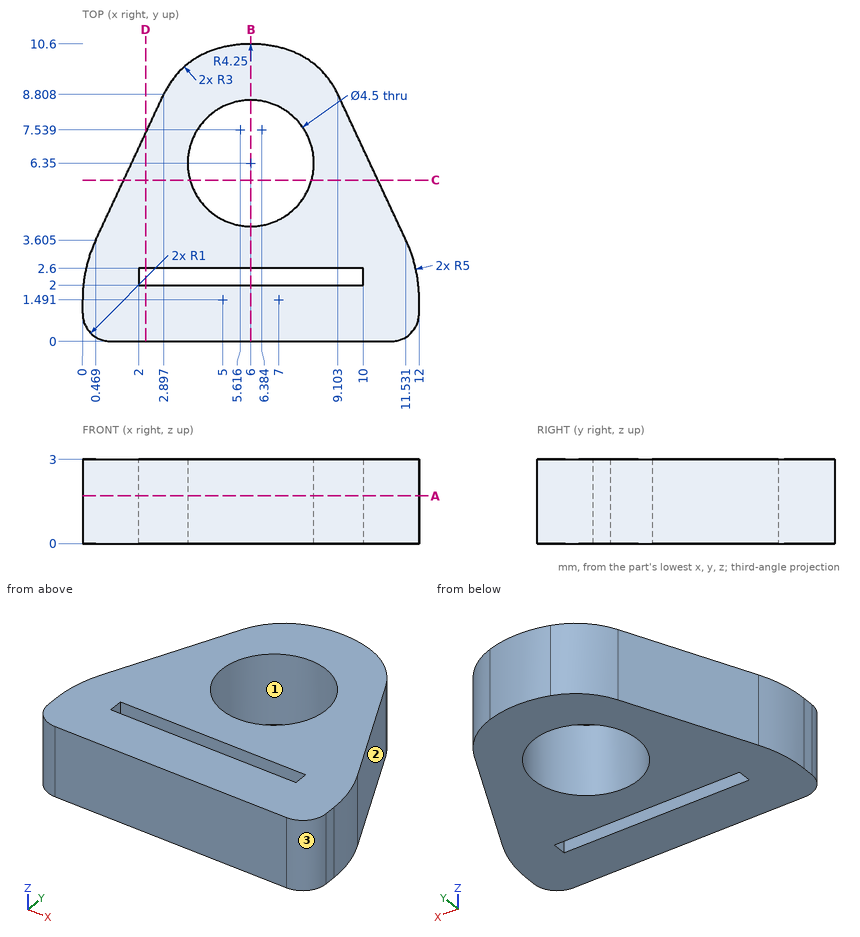
The drawing under review shows one solid part. Ordinate dimensions are in mm from its lowest x, y, z. Give positions to 0.01 mm unless a question says otherwise; leave off trailing zeros. Write each loop counter-clockwise with the first axis right and the second up, starting at its lowest first coordinate (ties: lowest second). Pieces come first, ordered by that corner, then holes. Notation, with made-up numbers: (-0.5, 32) -> (10.5, 32) arc R18 cw to (10.5, 40) -> close; hole circle Ø7 at (25, -14). An arc over 180 degrees is marked (long way). Put each result on its own line as item: value.
(1) We need section D-D, the plane x = 2.25. Give the boundary of the cut face in (y, z).
Results are:
outline: (0, 0) -> (2, 0) -> (2, 3) -> (0, 3) -> close; (2.6, 0) -> (7.42, 0) -> (7.42, 3) -> (2.6, 3) -> close
(2) We need section A-A, the plane z = 1.7. State how many separate pieces and enclosed holes the cut face has.
Results are:
separate pieces: 1
enclosed holes: 2
(3) To check wall thickness, follow probe 1 along Y at (x, z) = (6, 1.2); probe 2 along Y at (x, z) = (4.25, 0.65) (1 decimal); probe 3 along X at (y, z) = (7.25, 0.6). State the ranges of each line that lie inside material, in increasing order. Write a range as from..to.
Results are:
probe 1: 0..2, 2.6..4.1, 8.6..10.6
probe 2: 0..2, 2.6..4.9, 7.8..10.2
probe 3: 2.17..3.94, 8.06..9.83
(4) We need section B-B, the plane x = 6. Give the boundary of the cut face in (y, z), and give its area (3 significant figures).
Results are:
outline: (0, 0) -> (2, 0) -> (2, 3) -> (0, 3) -> close; (2.6, 0) -> (4.1, 0) -> (4.1, 3) -> (2.6, 3) -> close; (8.6, 0) -> (10.6, 0) -> (10.6, 3) -> (8.6, 3) -> close
area: 16.5 mm²
(5) We need section C-C, the plane y = 5.75. Give the boundary of the cut face in (x, z), and give its area (3 significant figures).
Results are:
outline: (1.47, 0) -> (3.83, 0) -> (3.83, 3) -> (1.47, 3) -> close; (8.17, 0) -> (10.53, 0) -> (10.53, 3) -> (8.17, 3) -> close
area: 14.2 mm²
(6) For pin 1 Ø1.5 at (x, z) = (10.5, 1.5) entering from +Y; pin 2 Ø1 at (y, z) = (3, 0.5) entering from -X, all flat-tipped, find the tip position at first contact; note any pin that passes through.
Results are:
pin 1: y = 7.42
pin 2: x = 0.1
(7) The part is to be moulded in two halves that separate along Y. For the marked faces 1, 2 and 3, say which applies: pulls with the +Y half, pulls with the -Y half, needs draft (parallel to the pull), parting line crosses it, or undercut.
Results are:
face 1: undercut
face 2: pulls with the +Y half
face 3: pulls with the -Y half
